```python
from build123d import *

# Parameters (mm, degrees)
SKETCH_1_W         = 50
SKETCH_1_H         = 162
BLOCKEXTRUDE_DEPTH = 70
FILLET_2_R         = 3
SHELL_START        = 3
SHELL_1_OUTLINE_W  = 159
SHELL_1_OUTLINE_H  = 64
SHELL_1_DEPTH      = 44
SKETCH_2_R         = 4.1
CABLE_ENTRY_DEPTH  = 184.423008371


# Read off the part's stored shape, not the designer's step: 抽壳1
with BuildPart() as part:
    # 草图1 → BlockExtrude (new body)
    with BuildSketch(Plane.XY):
        with Locations((25, 81)):
            Rectangle(SKETCH_1_W, SKETCH_1_H)
    extrude(amount=BLOCKEXTRUDE_DEPTH)

    # Fillet 2
    fillet_2_edges = [part.edges().sort_by_distance(p)[0] for p in [
        (50, 81, 70),
        (0, 81, 70),
        (50, 81, 0),
        (0, 81, 0),
    ]]
    fillet(fillet_2_edges, radius=FILLET_2_R)

    # 抽壳1 outline → 抽壳1 (cut)
    with BuildSketch(Plane.YZ.offset(SHELL_START)):
        with Locations((82.5, 35)):
            Rectangle(SHELL_1_OUTLINE_W, SHELL_1_OUTLINE_H)
    extrude(amount=SHELL_1_DEPTH, mode=Mode.SUBTRACT)

    # 草图2 → Cable_entry (cut, through all)
    with BuildSketch(Plane(origin=(0, 0, 0), x_dir=(-1, 0, 0), z_dir=(0, 0, -1))):
        with Locations((-25, 77)):
            Circle(SKETCH_2_R)
    extrude(amount=-CABLE_ENTRY_DEPTH, mode=Mode.SUBTRACT)


solid = part.part
```
Design review of the part built by this model. Coordinates are the model's own, in mm. A direction names the side the tool comes from. Coordinates: 2 decimals unless noted, no trailing zeros. Order: outer loops, then holes, each group sorted by start corner. A loop starts at its lowest first (then second) coordinate and runs counter-clockwise, first axis right, second up. Notation, with made-up numbers: M 31.5,25.25 L 40.5,25.25 A10 cw 40.5,31.25 Z; hole C 43,10 d7. An arc over 180 degrees is marked long. Answer as a JSON object with one key per item and string values. Group by question number.
1) Add section C-C, the plane z = 7.5. Write out the cut boundary in (x, y).
2) Tool access review of faces 1 (the flat face through (47, 81, 35)), 2 (the cylindrical face through (25.534, 81.065, 1.479)): name each direction out of +Z, -Z, +X, -X, +Y, -Y from which nothing blocks a thin tool from reaching the whole face with its end or side.
3) Add section B-B, the plane x = 25. Write out the cut boundary in (y, z).
4) Wall thickness on L1, parallel to X at y = 49, z = 38; L2, parallel to Z at x = 39.5, y = 72; L3, parallel to Y at x = 25, z = 2: over which ranges is each line inside the solid? List them lowest first.
5) Add section A-A, the plane y = 77. Write out the cut boundary in (x, z), then the cut area to 3 significant figures.
6) For pin 1 (8 mm diameter, centred on x = 39.5, z = 20.5, fed in from +Y); pin 2 (7.5 mm diameter, centred on x = 25, y = 77, fed in from +Z), all flat-tipped, find the tip position at first contact; note any pin that passes through.
7) Add section D-D, the plane x = 12. Write out the cut boundary in (y, z), then the cut area to 3 significant figures.
8) Mouldability with a two-part tool opening along Z and no side actions: class faces 3 (the flat face through (3, 81, 35)), 4 (the flat face through (25, 82, 70)), 5 (the flat face through (25, 0, 35)) as pulls with the +Z half, pulls with the -Z half, needs draft (parallel to the pull), parting line crosses it, or undercut.
Computed values:
{
 "1": {"outline": "M 0,0 L 50,0 L 50,162 L 47,162 L 47,3 L 3,3 L 3,162 L 0,162 Z"},
 "2": {"face 1": "+Y", "face 2": "+Z, -Z"},
 "3": {"outline": "M 0,0 L 72.9,0 L 72.9,3 L 3,3 L 3,67 L 72.9,67 L 72.9,70 L 0,70 Z; M 81.1,0 L 162,0 L 162,3 L 81.1,3 Z; M 81.1,67 L 162,67 L 162,70 L 81.1,70 Z"},
 "4": {"L1": "x = 0 to 3, 47 to 50", "L2": "z = 0 to 3, 67 to 70", "L3": "y = 0 to 72.9, 81.1 to 162"},
 "5": {"outline": "M 0,3 A3 ccw 3,0 L 20.9,0 L 20.9,3 L 3,3 L 3,67 L 20.9,67 L 20.9,70 L 3,70 A3 ccw 0,67 Z; M 29.1,0 L 47,0 A3 ccw 50,3 L 50,67 A3 ccw 47,70 L 29.1,70 L 29.1,67 L 47,67 L 47,3 L 29.1,3 Z", "area": "627 mm^2"},
 "6": {"pin 1": "stops at y = 3", "pin 2": "passes through"},
 "7": {"outline": "M 0,0 L 162,0 L 162,3 L 3,3 L 3,67 L 162,67 L 162,70 L 0,70 Z", "area": "1,160 mm^2"},
 "8": {"face 3": "undercut", "face 4": "pulls with the +Z half", "face 5": "needs draft"}
}
